Check sheet for the modelled part. Datum: model origin and axes. Units: mm. A direction names the side the tool comes from. Give positions to 0.01 mm unless a question says otherwise; leave off trailing zeros. Order: outer loops, then holes, each group sorted by start corner. A loop starts at its lowest first (then second) coordinate and runs counter-clockwise, first axis right, second up.
```python
from build123d import *

# Parameters (mm, degrees)
SKETCH_2_W           = 38
SKETCH_2_H           = 31
SKETCH_3_R           = 9.5
CUT_EXTRUDE_1_DEPTH  = 321.526909947
SKETCH_4_R           = 9.5
CUT_EXTRUDE_2_DEPTH  = 321.526909947
SKETCH_5_R           = 9.5
CUT_EXTRUDE_3_DEPTH  = 321.526909947
SKETCH_6_R           = 9.5
CUT_EXTRUDE_4_DEPTH  = 321.526909947
SKETCH_7_R           = 9.5
CUT_EXTRUDE_5_DEPTH  = 321.526909947
SKETCH_8_R           = 9.5
CUT_EXTRUDE_6_DEPTH  = 321.526909947
SKETCH_9_R           = 9.5
CUT_EXTRUDE_7_DEPTH  = 321.526909947
SKETCH_10_R          = 9.5
CUT_EXTRUDE_8_DEPTH  = 321.526909947
SKETCH_11_R          = 9.5
CUT_EXTRUDE_9_DEPTH  = 321.526909947
SKETCH_12_R          = 9.5
CUT_EXTRUDE_10_DEPTH = 321.526909947
SKETCH_13_R          = 9.5
CUT_EXTRUDE_11_DEPTH = 321.526909947
SKETCH_14_R          = 9.5
CUT_EXTRUDE_12_DEPTH = 321.526909947


with BuildPart() as part:
    # Эскиз1 → Повернуть1 (revolve)
    with BuildSketch(Plane.XY, mode=Mode.PRIVATE) as revolve_1_sk:
        Polygon((0, 0), (265, 0), (265, 127.5), (239, 127.5), (239, 100), (239, 95), (220, 95), (220, 94), (200, 94), (144, 65.5), (70, 65.5), (25, 41), (3, 41), (3, 45), (0, 45), align=None)
    revolve(revolve_1_sk.sketch.rotate(Axis((0, 0, 0), (1, 0, 0)), 90), axis=Axis((0, 0, 0), (1, 0, 0)))

    # Эскиз2 → Вырез-Повернуть1 (revolve, cut)
    with BuildSketch(Plane.XY, mode=Mode.PRIVATE) as cut_revolve_1_sk:
        with Locations((19, 15.5)):
            Rectangle(SKETCH_2_W, SKETCH_2_H)
    revolve(cut_revolve_1_sk.sketch.rotate(Axis((0, 0, 0), (1, 0, 0)), 90), axis=Axis((0, 0, 0), (1, 0, 0)), mode=Mode.SUBTRACT)

    # Эскиз3 → Вырез-Вытянуть1 (cut, through all)
    with BuildSketch(Plane(origin=(0, 0, 0), x_dir=(0, 0, -1), z_dir=(1, 0, 0))):
        with Locations((0, 113)):
            Circle(SKETCH_3_R)
    extrude(amount=CUT_EXTRUDE_1_DEPTH, mode=Mode.SUBTRACT)

    # Эскиз4 → Вырез-Вытянуть2 (cut, through all)
    with BuildSketch(Plane(origin=(0, 0, 0), x_dir=(0, 0, -1), z_dir=(1, 0, 0))):
        with Locations((-56.5, 97.860870628)):
            Circle(SKETCH_4_R)
    extrude(amount=CUT_EXTRUDE_2_DEPTH, mode=Mode.SUBTRACT)

    # Эскиз5 → Вырез-Вытянуть3 (cut, through all)
    with BuildSketch(Plane(origin=(0, 0, 0), x_dir=(0, 0, -1), z_dir=(1, 0, 0))):
        with Locations((-97.860870628, 56.5)):
            Circle(SKETCH_5_R)
    extrude(amount=CUT_EXTRUDE_3_DEPTH, mode=Mode.SUBTRACT)

    # Эскиз6 → Вырез-Вытянуть4 (cut, through all)
    with BuildSketch(Plane(origin=(0, 0, 0), x_dir=(0, 0, -1), z_dir=(1, 0, 0))):
        with Locations((-113, 0)):
            Circle(SKETCH_6_R)
    extrude(amount=CUT_EXTRUDE_4_DEPTH, mode=Mode.SUBTRACT)

    # Эскиз7 → Вырез-Вытянуть5 (cut, through all)
    with BuildSketch(Plane(origin=(0, 0, 0), x_dir=(0, 0, -1), z_dir=(1, 0, 0))):
        with Locations((-97.860870628, -56.5)):
            Circle(SKETCH_7_R)
    extrude(amount=CUT_EXTRUDE_5_DEPTH, mode=Mode.SUBTRACT)

    # Эскиз8 → Вырез-Вытянуть6 (cut, through all)
    with BuildSketch(Plane(origin=(0, 0, 0), x_dir=(0, 0, -1), z_dir=(1, 0, 0))):
        with Locations((-56.5, -97.860870628)):
            Circle(SKETCH_8_R)
    extrude(amount=CUT_EXTRUDE_6_DEPTH, mode=Mode.SUBTRACT)

    # Эскиз9 → Вырез-Вытянуть7 (cut, through all)
    with BuildSketch(Plane(origin=(0, 0, 0), x_dir=(0, 0, -1), z_dir=(1, 0, 0))):
        with Locations((0, -113)):
            Circle(SKETCH_9_R)
    extrude(amount=CUT_EXTRUDE_7_DEPTH, mode=Mode.SUBTRACT)

    # Эскиз10 → Вырез-Вытянуть8 (cut, through all)
    with BuildSketch(Plane(origin=(0, 0, 0), x_dir=(0, 0, -1), z_dir=(1, 0, 0))):
        with Locations((56.5, -97.860870628)):
            Circle(SKETCH_10_R)
    extrude(amount=CUT_EXTRUDE_8_DEPTH, mode=Mode.SUBTRACT)

    # Эскиз11 → Вырез-Вытянуть9 (cut, through all)
    with BuildSketch(Plane(origin=(0, 0, 0), x_dir=(0, 0, -1), z_dir=(1, 0, 0))):
        with Locations((97.860870628, -56.5)):
            Circle(SKETCH_11_R)
    extrude(amount=CUT_EXTRUDE_9_DEPTH, mode=Mode.SUBTRACT)

    # Эскиз12 → Вырез-Вытянуть10 (cut, through all)
    with BuildSketch(Plane(origin=(0, 0, 0), x_dir=(0, 0, -1), z_dir=(1, 0, 0))):
        with Locations((113, 0)):
            Circle(SKETCH_12_R)
    extrude(amount=CUT_EXTRUDE_10_DEPTH, mode=Mode.SUBTRACT)

    # Эскиз13 → Вырез-Вытянуть11 (cut, through all)
    with BuildSketch(Plane(origin=(0, 0, 0), x_dir=(0, 0, -1), z_dir=(1, 0, 0))):
        with Locations((97.860870628, 56.5)):
            Circle(SKETCH_13_R)
    extrude(amount=CUT_EXTRUDE_11_DEPTH, mode=Mode.SUBTRACT)

    # Эскиз14 → Вырез-Вытянуть12 (cut, through all)
    with BuildSketch(Plane(origin=(0, 0, 0), x_dir=(0, 0, -1), z_dir=(1, 0, 0))):
        with Locations((56.5, 97.860870628)):
            Circle(SKETCH_14_R)
    extrude(amount=CUT_EXTRUDE_12_DEPTH, mode=Mode.SUBTRACT)


solid = part.part
```
(1) Set-up check for faces 1 (the face through (19.266, -30.736, -4.036)), 2 (the face through (251.818, 2.854, -122.061)), 3 (the face through (27.185, 41.186, -9.146)): record each of +Z, -Z, +X, -X, +Y, -Y from which the full face is reachable in a straight line by a thin tool's end or side.
Response values:
face 1: -X
face 2: +X, -X
face 3: none
(2) Release check for a two-part mould opening along Y. For faces 4 (the face through (146.719, -20.09, 63.795)), 5 (the face through (239, -95, -10)), 6 (the face through (251.818, 100.714, 47.439)) record: released by +Y, released by -Y, zero draft, split by the parting line, or undercut.
Response values:
face 4: split by the parting line
face 5: zero draft
face 6: undercut
(3) Cross-section at D-D on x = 160. Enter the section's corners in (y, z), then the cut area to 3 significant figures.
Response values:
outline: circle Ø147.29 at (0, 0)
area: 17,000 mm2
(4) Material ranges on L1, parallel to Y at x = 259.75, z = 0; L2, parallel to Y at x = 24, z = 0; L3, parallel to Y at x = 252, z = 56.5, recorded low to high.
Response values:
L1: y = -127.5 to -122.5, -103.5 to 103.5, 122.5 to 127.5
L2: y = -41 to -31, 31 to 41
L3: y = -114.3 to -107.36, -88.36 to 88.36, 107.36 to 114.3
(5) Cross-section at A-A on y = 113. Enter the section's corners in (x, z).
Response values:
outline: (239, -59.05) - (265, -59.05) - (265, -9.5) - (239, -9.5) - close; (239, 9.5) - (265, 9.5) - (265, 59.05) - (239, 59.05) - close
(6) Cross-section at B-B on z = 0. Count the separate pieces of the cut face and the enclosed holes in it, then the cut area to 3 significant figures.
Response values:
separate pieces: 3
enclosed holes: 0
area: 36,100 mm2
(7) Gauge pin test, flat ends, axial feed: pin 1 Ø8 at (x, z) = (203, -65.5) entering from +Y; pin 2 Ø5 at (x, z) = (66, -23.5) entering from -Y. Record the tip position at first contact, or that the pin passes through.
Response values:
pin 1: stops at y = 71.09
pin 2: stops at y = -60.54
